from build123d import *

# Parameters (mm, degrees)
SKETCH1_W           = 177.8
SKETCH1_H           = 3.175
BOSS_EXTRUDE1_DEPTH = 3.175
SKETCH2_R           = 2.54
CUT_EXTRUDE1_DEPTH  = 4.175


with BuildPart() as part:
    # Sketch1 → Boss-Extrude1 (new body)
    with BuildSketch(Plane.XY):
        Polygon((228.6, -6.35), (228.6, -3.175), (254, -3.175), (254, 301.625), (203.2, 301.625), (203.2, 307.975), (152.4, 307.975), (152.4, 301.625), (101.6, 301.625), (101.6, 307.975), (50.8, 307.975), (50.8, 301.625), (0, 301.625), (0, -3.175), (25.4, -3.175), (25.4, -6.35), align=None)
        with Locations((127, 287.3375)):
            Rectangle(SKETCH1_W, SKETCH1_H, mode=Mode.SUBTRACT)
    extrude(amount=BOSS_EXTRUDE1_DEPTH)

    # Sketch2 → Cut-Extrude1 (cut, through all)
    with BuildSketch(Plane(origin=(0, 0, 0), x_dir=(-1, 0, 0), z_dir=(0, 0, -1))):
        with Locations((-234.063292103, 250.825)):
            Circle(SKETCH2_R)
        with Locations((-234.063292103, 98.425)):
            Circle(SKETCH2_R)
    extrude(amount=-CUT_EXTRUDE1_DEPTH, mode=Mode.SUBTRACT)


solid = part.part
CAD build for the part. Positions are in the model's coordinates, mm. Round coordinates to 2 decimals unless told otherwise and drop trailing zeros. Write each loop counter-clockwise with the first axis right and the second up, starting at its lowest first coordinate (ties: lowest second). Pieces come first, ordered by that corner, then holes.
(1) Slice it at A-A, the plane z = 1. Write the cut outline in (x, y) (3 decimals), and give its area (3 significant figures).
(2) Drop flat-ended pins along their axis: P1, Ø1.6, axis at x = 12, z = 1.5, coming from the -Y side (3 decimals); P2, Ø1, axis at x = 136.5, z = 1.5, coming from the +Y side (3 decimals); P3, Ø3, axis at x = 234.06, y = 98.42, coming from the +Z side; P4, Ø1, axis at y = 304.5, z = 2, coming from the +X side. Give the stop position or say it passes through.
(3) Probe line 1 along Y through (x, z) = (138, 1.25) (3 decimals); line 2 along Y through (x, z) = (225, 1.2) (3 decimals); line 3 along Y through (x, z) = (98.5, 1.8) (3 decimals). List the from-to ranges inside material, lowest first.
From the geometry:
1. outline: (0, -3.175) - (25.4, -3.175) - (25.4, -6.35) - (228.6, -6.35) - (228.6, -3.175) - (254, -3.175) - (254, 301.625) - (203.2, 301.625) - (203.2, 307.975) - (152.4, 307.975) - (152.4, 301.625) - (101.6, 301.625) - (101.6, 307.975) - (50.8, 307.975) - (50.8, 301.625) - (0, 301.625) - close; hole (38.1, 285.75) - (215.9, 285.75) - (215.9, 288.925) - (38.1, 288.925) - close; hole circle Ø5.08 at (234.063, 98.425); hole circle Ø5.08 at (234.063, 250.825)
1. area: 78,100 mm2
2. P1: stops at y = -3.175
2. P2: stops at y = 301.625
2. P3: passes through
2. P4: stops at x = 203.2
3. line 1: y = -6.35 to 285.75, 288.925 to 301.625
3. line 2: y = -6.35 to 301.625
3. line 3: y = -6.35 to 285.75, 288.925 to 307.975
